The model under review builds one solid part; all positions refer to its coordinate system, in mm. A direction names the side the tool comes from. Round coordinates to 2 decimals unless told otherwise and drop trailing zeros. Loops run counter-clockwise (first coordinate to the right, second up) from the corner with the lowest first, then second, coordinate; pieces in that order, holes last. Notation, with made-up numbers: M 68,84 L 102,84 A24 cw 102,104 Z; hole C 17,21 d3. An arc over 180 degrees is marked long. Answer in a Markdown table with one row per item. Add a question column.
from build123d import *

# Parameters (mm, degrees)
SKETCH_R            = 5.5
PAD_DEPTH           = 4
POCKET_DEPTH        = 1
SKETCH006_W         = 11
SKETCH006_H         = 6.5
PAD001_DEPTH        = 3
PAD002_DEPTH        = 3
SKETCH004_R         = 1
MIRROREDSKETCH003_R = 1
SKETCH008_R         = 2.5
POCKET001_DEPTH     = 3
FILLET_R            = 1


with BuildPart() as part:
    # Sketch → Pad (new body, symmetric)
    with BuildSketch(Plane.XY):
        Circle(SKETCH_R)
    extrude(amount=PAD_DEPTH, both=True)

    # Sketch002 → Pocket (cut, symmetric)
    with BuildSketch(Plane.XY):
        with BuildLine():
            ThreePointArc((-5.291503, -1.5), (0, -5.5), (5.291503, -1.5))
            add(Edge.make_bspline(
                [(-5.291503, -1.5), (0, -4.166667), (5.291503, -1.5)],
                knots=[3.785094, 3.785094, 3.785094, 5.639684, 5.639684, 5.639684], degree=2, weights=[1, 0.6, 1]))
        make_face()
        with BuildLine():
            ThreePointArc((5.291503, 1.5), (0, 5.5), (-5.291503, 1.5))
            add(Edge.make_bspline(
                [(5.291503, 1.5), (0, 4.166667), (-5.291503, 1.5)],
                knots=[0.643501, 0.643501, 0.643501, 2.498092, 2.498092, 2.498092], degree=2, weights=[1, 0.6, 1]))
        make_face()
    extrude(amount=POCKET_DEPTH, both=True, mode=Mode.SUBTRACT)

    # Sketch006 (on DatumPlane) → Pad001 (join)
    with BuildSketch(Plane.XY.offset(4)):
        with Locations((0, -3.25)):
            Rectangle(SKETCH006_W, SKETCH006_H)
    extrude(amount=-PAD001_DEPTH)

    # Sketch007 (on DatumPlane) → Pad002 (join)
    with BuildSketch(Plane(origin=(0, -6.5, 4), x_dir=(1, 0, 0), z_dir=(0, -0.258819, 0.965926))):
        with BuildLine():
            Line((-5.5, 0), (-4.48051, -10.918363))
            ThreePointArc((-4.48051, -10.918363), (0, -15), (4.48051, -10.918363))
            Line((4.48051, -10.918363), (5.5, 0))
            Line((5.5, 0), (-5.5, 0))
        make_face()
    extrude(amount=-PAD002_DEPTH)

    # SubtractivePipe: sweep along a path in MirroredSketch002
    with BuildLine(Plane.XZ) as subtractivepipe_path:
        ThreePointArc((-5.5, 0), (-2.671573, 1.171573), (-1.5, 4))
    # Sketch004 (on DatumPlane) → SubtractivePipe (sweep, cut)
    with BuildSketch(Plane.XY.offset(4)):
        with Locations((-1.5, 0)):
            Circle(SKETCH004_R)
    sweep(path=subtractivepipe_path.line, mode=Mode.SUBTRACT)

    # SubtractivePipe001: sweep along a path in Sketch003
    with BuildLine(Plane.XZ) as subtractivepipe001_path:
        ThreePointArc((1.5, 4), (2.671573, 1.171573), (5.5, 0))
    # MirroredSketch003 → SubtractivePipe001 (sweep, cut)
    with BuildSketch(Plane.XY.offset(4)):
        with Locations((1.5, 0)):
            Circle(MIRROREDSKETCH003_R)
    sweep(path=subtractivepipe001_path.line, mode=Mode.SUBTRACT)

    # Sketch008 (on DatumPlane) → Pocket001 (cut)
    with BuildSketch(Plane(origin=(0, -6.5, 4), x_dir=(1, 0, 0), z_dir=(0, -0.258819, 0.965926))):
        with Locations((0, -10.5)):
            Circle(SKETCH008_R)
    extrude(amount=-POCKET001_DEPTH, mode=Mode.SUBTRACT)

    # Fillet
    fillet_edges = [part.edges().sort_by_distance(p)[0] for p in [
        (0, 5.5, -1),
        (0, 5.5, 1),
        (0, -5.5, -1),
    ]]
    fillet(fillet_edges, radius=FILLET_R)


solid = part.part
1. Take a section at C-C, the plane z = -3.5. State the section outline as (x, y) points, and give its area (3 significant figures).
2. Take a section at B-B, the plane z = 0.5. State how many separate pieces and enclosed holes the cut face has, and give its area (3 significant figures).
3. Mouldability with a two-part tool opening along Y and no side actions: class faces 4 (the flat face through (-5.5, -3, 3)), 5 (the cylindrical face through (-0.542, -18.617, -0.778)), 6 (the flat face through (-0.08, -12.03, 2.52)) as released by +Y, released by -Y, zero draft, split by the parting line, or undercut.
4. To check wall thickness, follow probe 1 along Z at (x, y) = (2.5, -3.75); probe 2 along X at (y, z) = (1.5, -2.5); probe 3 along X at (y, z) = (-17.75, -1.5). State the ranges of each line that lie inside material, in increasing order.
5. Machinability: for faces 1 (the cylindrical face through (-0.716, 5.453, -2.611)), 2 (the flat face through (-0.076, -11.492, -0.444)), 3 (the flat face through (0, 0, 4)), which of the approach directions +Z, -Z, +X, -X, +Y, -Y give a long, thin tool a straight path to every point of the face, cutting with its end or side? Answer none if there is none.
6. For pin 1 Ø1 at (y, z) = (3, 2) entering from +X; pin 2 Ø5 at (x, y) = (2, -8) entering from -Z; pin 3 Ø1 at (x, y) = (-4.5, -13.5) entering from +Z, all flat-tipped, find the tip position at first contact; note any pin that passes through.
7. Take a section at A-A, the plane y = 0.5. State the section outline as (x, z) points, and give its area (3 significant figures).
Check sheet entries:
| question | item | result |
|---|---|---|
| 1 | outline | C 0,0 d11 |
| 1 | area | 95.0 mm^2 |
| 2 | separate pieces | 2 |
| 2 | enclosed holes | 1 |
| 2 | area | 123 mm^2 |
| 3 | face 4 | zero draft |
| 3 | face 5 | undercut |
| 3 | face 6 | released by -Y |
| 4 | probe 1 | z = -4 to -1, 1 to 4 |
| 4 | probe 2 | x = -5.29 to 5.29 |
| 4 | probe 3 | x = -4.13 to -1.75, 1.75 to 4.13 |
| 5 | face 1 | -Z |
| 5 | face 2 | -Z, +X, -X |
| 5 | face 3 | +Z, +X, -X, +Y, -Y |
| 6 | pin 1 | stops at x = 4.9 |
| 6 | pin 2 | stops at z = -0.18 |
| 6 | pin 3 | stops at z = 2.26 |
| 7 | outline | M -5.48,-4 L 5.48,-4 L 5.48,-0.87 A4.87 cw 0.63,4 L -0.63,4 A4.87 cw -5.48,-0.87 Z; M -5.48,0.87 A3.13 ccw -2.37,4 L -5.48,4 Z; M 2.37,4 A3.13 ccw 5.48,0.87 L 5.48,4 Z |
| 7 | area | 65.9 mm^2 |
